Check sheet for the modelled part. Datum: model origin and axes. Units: mm. Face numbers are marked on the shaded views. Give positions to 0.01 mm unless a question says otherwise; leave off trailing zeros. Order: outer loops, then holes, each group sorted by start corner. A loop starts at its lowest first (then second) coordinate and runs counter-clockwise, first axis right, second up.
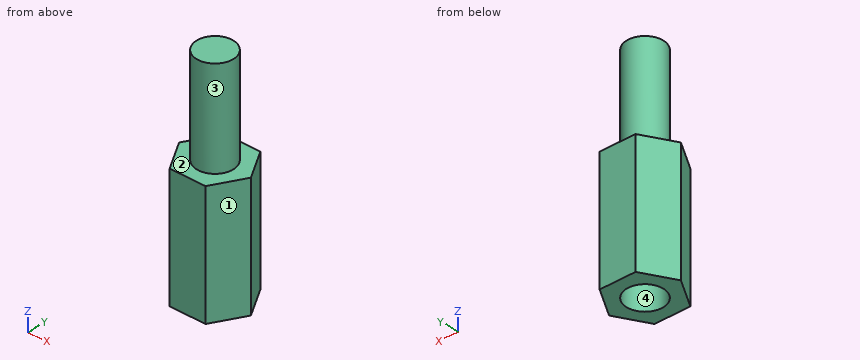
```python
from build123d import *

# Parameters (mm, degrees)
BOSS_EXTRU_1_DEPTH      = 10
ESQUISSE2_R             = 1.5
BOSS_EXTRU_2_DEPTH      = 8
ESQUISSE3_R             = 1.5
ENL_V_MAT_EXTRU_1_DEPTH = 8


with BuildPart() as part:
    # Esquisse1 → Boss.-Extru.1 (new body)
    with BuildSketch(Plane.XY):
        Polygon((2.886751346, 0), (1.443375673, 2.5), (-1.443375673, 2.5), (-2.886751346, 0), (-1.443375673, -2.5), (1.443375673, -2.5), align=None)
    extrude(amount=BOSS_EXTRU_1_DEPTH)

    # Esquisse2 → Boss.-Extru.2 (add)
    with BuildSketch(Plane.XY.offset(10)):
        Circle(ESQUISSE2_R)
    extrude(amount=BOSS_EXTRU_2_DEPTH)

    # Esquisse3 → Enlèv. mat.-Extru.1 (cut)
    with BuildSketch(Plane(origin=(0, 0, 0), x_dir=(-1, 0, 0), z_dir=(0, 0, -1))):
        with Locations(Location((0, 0, 0), (0, 0, 180))):
            Circle(ESQUISSE3_R)
    extrude(amount=-ENL_V_MAT_EXTRU_1_DEPTH, mode=Mode.SUBTRACT)


solid = part.part
```
(1) Thickness scan on L1, parallel to Y at x = 0, z = 2; L2, parallel to Z at x = 0.4, y = 0.1; L3, parallel to Z at x = 2.2, y = 0.7. Record the ranges inside material, lowest first.
(2) Sectioned sample at B-B (x = 0). Enter the section's corners in (y, z), plus the area to 3 significant figures.
(3) Sectioned sample at A-A (z = 6.25). Enter the section's corners in (x, y).
(4) Sectioned sample at C-C (y = 1). Enter the section's corners in (x, z), plus the area to 3 significant figures.
(5) Go/stop test with a flat-tipped pin: P1, Ø1.5, axis at x = 0.5, y = -0.5, coming from the -Z side. Record where the tip stops, or that it passes through.
(6) Sectioned sample at D-D (z = 8.5). Enter the section's corners in (x, y), plus the area to 3 significant figures.
(7) Release check for a two-part mould opening along Y. For the marked faces 1, 2, 3 and 4 record: released by +Y, released by -Y, zero draft, split by the parting line, or undercut.
Values follow:
1. L1: y = -2.5 to -1.5, 1.5 to 2.5
1. L2: z = 8 to 18
1. L3: z = 0 to 10
2. outline: (-2.5, 0) - (-1.5, 0) - (-1.5, 8) - (1.5, 8) - (1.5, 0) - (2.5, 0) - (2.5, 10) - (1.5, 10) - (1.5, 18) - (-1.5, 18) - (-1.5, 10) - (-2.5, 10) - close
2. area: 50.0 mm2
3. outline: (-2.89, 0) - (-1.44, -2.5) - (1.44, -2.5) - (2.89, 0) - (1.44, 2.5) - (-1.44, 2.5) - close; hole circle Ø3 at (0, 0)
4. outline: (-2.31, 0) - (-1.12, 0) - (-1.12, 8) - (1.12, 8) - (1.12, 0) - (2.31, 0) - (2.31, 10) - (1.12, 10) - (1.12, 18) - (-1.12, 18) - (-1.12, 10) - (-2.31, 10) - close
4. area: 46.2 mm2
5. P1: stops at z = 8
6. outline: (-2.89, 0) - (-1.44, -2.5) - (1.44, -2.5) - (2.89, 0) - (1.44, 2.5) - (-1.44, 2.5) - close
6. area: 21.7 mm2
7. face 1: released by -Y
7. face 2: zero draft
7. face 3: split by the parting line
7. face 4: undercut
